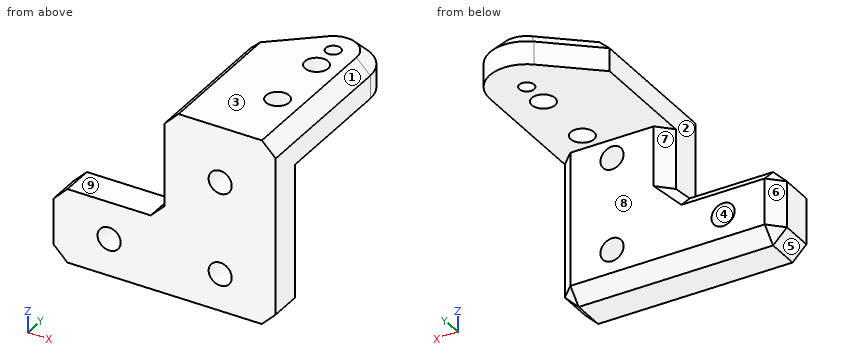
```python
from build123d import *

# Parameters (mm, degrees)
RESSALTO_EXTRUS_O1_DEPTH                = 20
ESBO_O2_W                               = 16
ESBO_O2_H                               = 16
CORTE_EXTRUS_O1_DEPTH                   = 20
CORTE_EXTRUS_O2_DEPTH                   = 34.120990323
CHANFRO2_SIZE                           = 1.5
FURO_ROSCADO_DE_M21_D                   = 1.6
ESBO_O8_W                               = 8
ESBO_O8_H                               = 5
RESSALTO_EXTRUS_O2_DEPTH                = 12
CHANFRO3_SIZE                           = 1.5
FURO_ROSCADO_DE_M31_D                   = 2.5
FURO_ROSCADO_DE_M31_DEPTH               = 8.5
FURO_ROSCADO_DE_M31_TIP                 = 0.751075774
BROCA_DE_ROSQUEAR_PARA_TARRAXA_DE_M31_D = 2.5


with BuildPart() as part:
    # Esboço1 → Ressalto-extrusão1 (new body)
    with BuildSketch(Plane.XY):
        with BuildLine():
            Line((0, 0), (0, 12))
            Line((0, 12), (9.400080843, 20.039805977))
            ThreePointArc((9.400080843, 20.039805977), (13.673368365, 20.633158174), (16, 17))
            Line((16, 17), (16, 4))
            Line((16, 4), (16, 0))
            Line((16, 0), (0, 0))
        make_face()
    extrude(amount=RESSALTO_EXTRUS_O1_DEPTH)

    # Esboço2 → Corte-extrusão1 (cut)
    with BuildSketch(Plane(origin=(16, 0, 0), x_dir=(0, 0, -1), z_dir=(1, 0, 0))):
        with Locations((-8, 13)):
            Rectangle(ESBO_O2_W, ESBO_O2_H)
    extrude(amount=-CORTE_EXTRUS_O1_DEPTH, mode=Mode.SUBTRACT)

    # Esboço3 → Corte-extrusão2 (cut, through all)
    with BuildSketch(Plane.XY.offset(20)):
        Polygon((0, 0), (4, 0), (4, 15.42116461), (0, 12), align=None)
    extrude(amount=-CORTE_EXTRUS_O2_DEPTH, mode=Mode.SUBTRACT)

    # Chanfro2
    chanfro2_edges = [part.edges().sort_by_distance(p)[0] for p in [
        (13.673368365, 20.633158174, 20),
        (6.700040421, 17.730485293, 20),
        (4, 7.710582305, 20),
        (16, 8.5, 20),
    ]]
    chamfer(chanfro2_edges, length=CHANFRO2_SIZE)

    # Furo roscado de M21 (through all)
    with Locations(Plane(origin=(12, 17, 20), x_dir=(1, 0, 0), z_dir=(0, 0, 1))):
        with Locations((0, 0)):
            Hole(FURO_ROSCADO_DE_M21_D / 2)

    # Esboço8 → Ressalto-extrusão2 (add)
    with BuildSketch(Plane.ZY.offset(-4)):
        with Locations((4, 2.5)):
            Rectangle(ESBO_O8_W, ESBO_O8_H)
    extrude(amount=RESSALTO_EXTRUS_O2_DEPTH)

    # Chanfro3
    chanfro3_edges = [part.edges().sort_by_distance(p)[0] for p in [
        (-2, 5, 8),
        (-8, 2.5, 0),
        (-8, 2.5, 8),
        (-8, 5, 4),
        (4, 5, 0),
        (16, 5, 8),
        (16, 2.5, 0),
        (4, 5, 12),
        (4, 2.5, 8),
    ]]
    chamfer(chanfro3_edges, length=CHANFRO3_SIZE)

    # Furo roscado de M31
    with Locations(Plane(origin=(-2, 0, 4), x_dir=(0, 0, -1), z_dir=(0, -1, 0))):
        with Locations((0, 0), (0, 12), (-10, 12)):
            Hole(FURO_ROSCADO_DE_M31_D / 2, depth=FURO_ROSCADO_DE_M31_DEPTH)
            with Locations((0, 0, -(FURO_ROSCADO_DE_M31_DEPTH + FURO_ROSCADO_DE_M31_TIP / 2))):  # 118° drill point
                Cone(0, FURO_ROSCADO_DE_M31_D / 2, FURO_ROSCADO_DE_M31_TIP, mode=Mode.SUBTRACT)

    # Broca de rosquear para tarraxa de M31 (through all)
    with Locations(Plane(origin=(12, 7, 20), x_dir=(1, 0, 0), z_dir=(0, 0, 1))):
        with Locations((0, 0), (0, 7)):
            Hole(BROCA_DE_ROSQUEAR_PARA_TARRAXA_DE_M31_D / 2)


solid = part.part
```
Can you work these out from the model? Positions are in its coordinate system, mm. Face numbers are marked on the shaded views. A direction names the side the tool comes from. Round coordinates to 2 decimals unless told otherwise and drop trailing zeros. Order: outer loops, then holes, each group sorted by start corner. A loop starts at its lowest first (then second) coordinate and runs counter-clockwise, first axis right, second up. Notation, with made-up numbers: (44, 18.5) -> (97, 18.5) arc R31 ccw to (97, 43.5) -> close; hole circle Ø6 at (51.5, 19.5). An arc over 180 degrees is marked (long way). Return JSON: item names as keys, results as strings. Group by question number.
1. If we section it at D-D, the plane z = 9: Write out the boundary of the cut face in (x, y), then the cut area to 4 significant figures.
2. We'd pull the mould along X, two halves only. Please class the marked faces 1, 2, 3 and 4: released by +X, released by -X, zero draft, split by the parting line, or undercut.
3. I need wall thicknesses on line 1 (Y direction, x = 12, z = 17.6); line 2 (X direction, y = 1.5, z = 4); line 3 (Y direction, x = 12, z = 19.1). Which ranges of each line are inside material? Lowest first, please. Write a range as [from, to].
4. Will these pins go through, and if not, where does the flat tip stop? pin 1 (3 mm diameter, centred on x = 5, y = 8, fed in from -Z); pin 2 (7 mm diameter, centred on x = 8.5, z = 9.5, fed in from +Y); pin 3 (4 mm diameter, centred on x = -1, y = 1, fed in from +Z).
5. If we section it at C-C, the plane x = -2: Write out the boundary of the cut face in (y, z), then the cut area to 4 significant figures.
6. If we section it at A-A, the plane z = 14: Write out the boundary of the cut face in (x, y).
7. If we section it at B-B, the plane z = 4.75: Write out the boundary of the cut face in (x, y).
8. Which directions (+Z, -Z, +X, -X, +Y, -Y) give clear straight access to the entire face, cutting with the end or side of a thin tool? Please do the marked faces 5, 6, 7, 8 and 9.
Output values:
{
 "1": {"outline": "(3.5, 0) -> (16, 0) -> (16, 3.5) -> (14.5, 5) -> (5, 5) -> (3.5, 3.5) -> close", "area": "60.25 mm²"},
 "2": {"face 1": "released by +X", "face 2": "released by -X", "face 3": "zero draft", "face 4": "undercut"},
 "3": {"line 1": "[0, 5.75], [8.25, 12.75], [15.25, 16.2], [17.8, 21]", "line 2": "[-8, -3.25], [-0.75, 8.75], [11.25, 16]", "line 3": "[0, 5.75], [8.25, 12.75], [15.25, 16.2], [17.8, 20.4]"},
 "4": {"pin 1": "z = 16", "pin 2": "y = 5", "pin 3": "z = 8"},
 "5": {"outline": "(0, 0) -> (3.5, 0) -> (5, 1.5) -> (5, 2.75) -> (0, 2.75) -> close; (0, 5.25) -> (5, 5.25) -> (5, 6.5) -> (3.5, 8) -> (0, 8) -> close", "area": "25.25 mm²"},
 "6": {"outline": "(4, 0) -> (8.75, 0) -> (8.75, 5) -> (5.5, 5) -> (4, 3.5) -> close; (11.25, 0) -> (16, 0) -> (16, 3.5) -> (14.5, 5) -> (11.25, 5) -> close"},
 "7": {"outline": "(-8, 0) -> (-3, 0) -> (-3, 5) -> (-6.5, 5) -> (-8, 3.5) -> close; (-1, 0) -> (9, 0) -> (9, 5) -> (-1, 5) -> close; (11, 0) -> (16, 0) -> (16, 3.5) -> (14.5, 5) -> (11, 5) -> close"},
 "8": {"face 5": "-Z, -X, +Y, -Y", "face 6": "+Z, -Z, -X, +Y", "face 7": "-X, +Y", "face 8": "-Z, +X, -X, +Y", "face 9": "+Z, -X, +Y, -Y"}
}
